Verification items for the finished model (mm, model axes). Coordinates: 2 decimals unless noted, no trailing zeros.
Q1. Cross-section at A-A, the plane z = 0.3. Count the separate pieces of the cut face and the enclosed holes in it, and give its area (3 significant figures).
Q2. Depth check by flat-ended pin: P1, Ø4.5, axis at x = 0, y = 225, coming from the +Z side; P2, Ø6.5, axis at x = 0, y = 325, coming from the -Z side. Enter the tip coordinate at first touch or a pass-through.
Q3. Thickness scan on line 1 (X direction, y = 325, z = 0.4). Record the ranges inside material, lowest first.
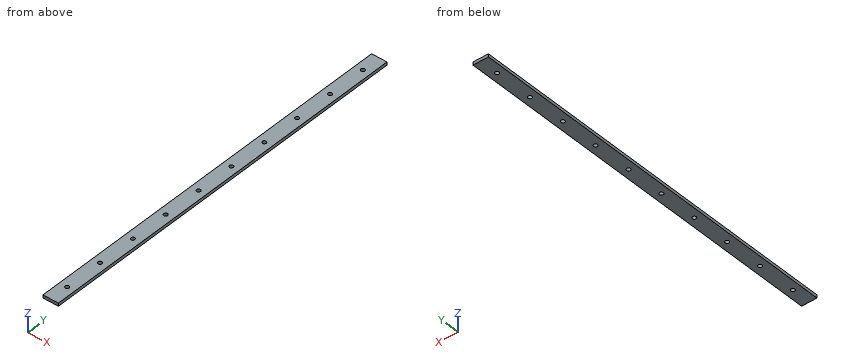
from build123d import *

# Parameters (mm, degrees)
SKETCH_1_W          = 20
SKETCH_1_H          = 4
EXTRUDE_1_DEPTH     = 500
SKETCH_2_R          = 2.5
CUT_EXTRUDE_1_DEPTH = 5


with BuildPart() as part:
    # Эскиз1 → Бобышка-Вытянуть1 (new body)
    with BuildSketch(Plane(origin=(0, 0, 0), x_dir=(1, 0, 0), z_dir=(0, 1, 0))):
        Rectangle(SKETCH_1_W, SKETCH_1_H)
    extrude(amount=EXTRUDE_1_DEPTH)

    # Эскиз2 → Вырез-Вытянуть1 (cut, through all)
    with BuildSketch(Plane.XY.offset(2)):
        with Locations((0, 25)):
            Circle(SKETCH_2_R)
        with Locations((0, 75)):
            Circle(SKETCH_2_R)
        with Locations((0, 125)):
            Circle(SKETCH_2_R)
        with Locations((0, 175)):
            Circle(SKETCH_2_R)
        with Locations((0, 225)):
            Circle(SKETCH_2_R)
        with Locations((0, 275)):
            Circle(SKETCH_2_R)
        with Locations((0, 325)):
            Circle(SKETCH_2_R)
        with Locations((0, 375)):
            Circle(SKETCH_2_R)
        with Locations((0, 425)):
            Circle(SKETCH_2_R)
        with Locations((0, 475)):
            Circle(SKETCH_2_R)
    extrude(amount=-CUT_EXTRUDE_1_DEPTH, mode=Mode.SUBTRACT)


solid = part.part
Check values:
1. separate pieces: 1
1. enclosed holes: 10
1. area: 9,800 mm2
2. P1: passes through
2. P2: stops at z = -2
3. line 1: x = -10 to -2.5, 2.5 to 10
